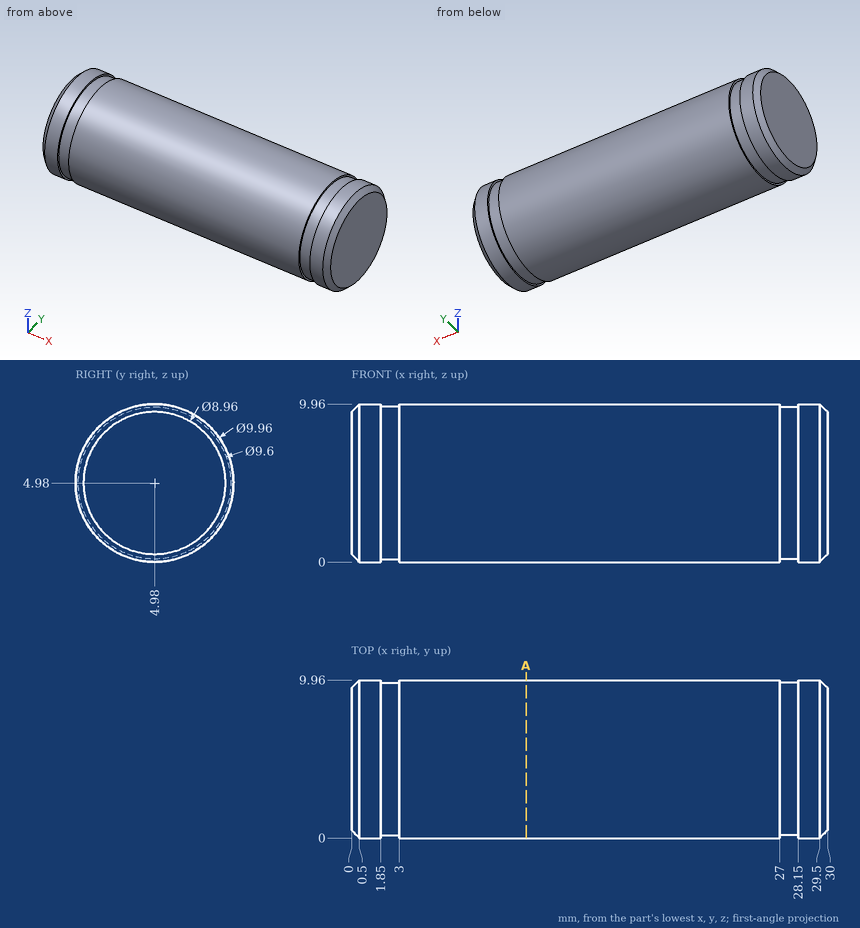
For this review, use the dimensioned drawing (mm, ordinates from the lowest corner) and the shaded views. Round coordinates to 2 decimals unless told otherwise and drop trailing zeros. Loops run counter-clockwise (first coordinate to the right, second up) from the corner with the lowest first, then second, coordinate; pieces in that order, holes last. Notation, with made-up numbers: M -8,77.5 L 7,77.5 A24 cw 7,105.5 Z; hole C -39,-9.75 d6. An arc over 180 degrees is marked long. Answer as a JSON object with one key per item and string values.
(1) To check wall thickness, follow line 1 along X through (y, z) = (1.75, 1.25); line 2 along Y through (x, z) = (19, 6.25); line 3 along Y through (x, z) = (9.5, 5.25). State the ranges of each line that lie inside material, in increasing order.
Resolved:
{"line 1": "0.45 to 1.85, 3 to 27, 28.15 to 29.55", "line 2": "0.16 to 9.8", "line 3": "0.01 to 9.95"}
(2) Take a section at A-A on x = 11. Give the boundary of the cut face in (y, z), and give its area (3 significant figures).
Resolved:
{"outline": "C 4.98,4.98 d9.96", "area": "77.9 mm²"}
(3) Clearance check with flat-ended pins moving along their axes: P1, Ø1.5, axis at x = 26.5, y = 3.5, coming from the +Z side; P2, Ø2, axis at x = 16.5, y = 7.5, coming from the -Z side; P3, Ø4, axis at x = 14.5, y = 8, coming from the -Z side. State where each tip first meets the part, or that it passes through.
Resolved:
{"P1": "z = 9.91", "P2": "z = 0.24", "P3": "z = 0.11"}
